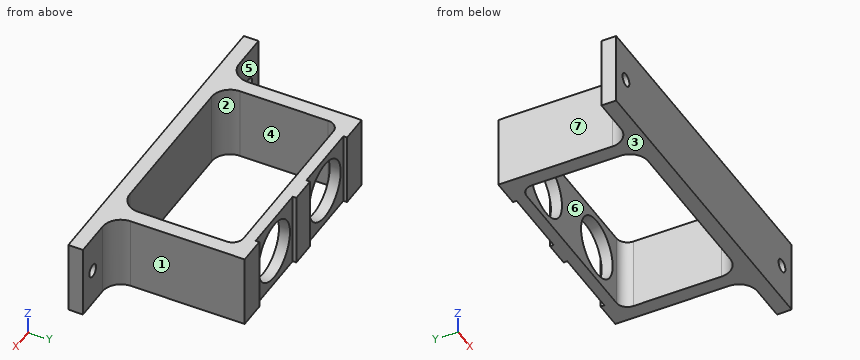
```python
from build123d import *

# Parameters (mm, degrees)
SKETCH_1_W          = 90
SKETCH_1_H          = 20
SKETCH_1_R          = 1.75
EXTRUDE_1_DEPTH     = 4
SKETCH_2_W          = 4
SKETCH_2_H          = 20
EXTRUDE_2_DEPTH     = 32
SKETCH_3_W          = 60
SKETCH_3_H          = 20
SKETCH_3_R          = 8.1
EXTRUDE_3_DEPTH     = 4
FILLET_1_R          = 5
FILLET_2_R          = 3
SKETCH_4_W          = 19
SKETCH_4_H          = 20
CUT_EXTRUDE_1_DEPTH = 1


with BuildPart() as part:
    # 草图1 → 凸台-拉伸1 (new body)
    with BuildSketch(Plane(origin=(0, 0, 0), x_dir=(1, 0, 0), z_dir=(0, 1, 0))):
        with Locations((45, 10)):
            Rectangle(SKETCH_1_W, SKETCH_1_H)
        with Locations(Location((85, 10, 0), (0, 0, 270))):
            Circle(SKETCH_1_R, mode=Mode.SUBTRACT)
        with Locations(Location((5, 10, 0), (0, 0, 90))):
            Circle(SKETCH_1_R, mode=Mode.SUBTRACT)
    extrude(amount=EXTRUDE_1_DEPTH)

    # 草图2 → 凸台-拉伸2 (add)
    with BuildSketch(Plane(origin=(0, 4, 0), x_dir=(1, 0, 0), z_dir=(0, 1, 0))):
        with Locations((17, 10)):
            Rectangle(SKETCH_2_W, SKETCH_2_H)
        with Locations((73, 10)):
            Rectangle(SKETCH_2_W, SKETCH_2_H)
    extrude(amount=EXTRUDE_2_DEPTH)

    # 草图3 → 凸台-拉伸3 (add)
    with BuildSketch(Plane(origin=(0, 36, 0), x_dir=(1, 0, 0), z_dir=(0, 1, 0))):
        with Locations((45, 10)):
            Rectangle(SKETCH_3_W, SKETCH_3_H)
        with Locations(Location((32, 10, 0), (0, 0, 270))):
            Circle(SKETCH_3_R, mode=Mode.SUBTRACT)
        with Locations(Location((58, 10, 0), (0, 0, 270))):
            Circle(SKETCH_3_R, mode=Mode.SUBTRACT)
    extrude(amount=EXTRUDE_3_DEPTH)

    # 圆角1
    fillet_1_edges = [part.edges().sort_by_distance(p)[0] for p in [
        (15, 4, -10),
        (19, 4, -10),
        (75, 4, -10),
        (71, 4, -10),
    ]]
    fillet(fillet_1_edges, radius=FILLET_1_R)

    # 圆角2
    fillet_2_edges = [part.edges().sort_by_distance(p)[0] for p in [
        (19, 36, -10),
        (71, 36, -10),
    ]]
    fillet(fillet_2_edges, radius=FILLET_2_R)

    # 草图4 → 切除-拉伸1 (cut)
    with BuildSketch(Plane(origin=(0, 40, 0), x_dir=(1, 0, 0), z_dir=(0, 1, 0))):
        with Locations((32, 10)):
            Rectangle(SKETCH_4_W, SKETCH_4_H)
        with Locations((58, 10)):
            Rectangle(SKETCH_4_W, SKETCH_4_H)
    extrude(amount=-CUT_EXTRUDE_1_DEPTH, mode=Mode.SUBTRACT)


solid = part.part
```
Geometry: final body of the model. Coordinates: model frame, mm. Face numbers are marked on the shaded views. A direction names the side the tool comes from. Coordinates: 2 decimals unless noted, no trailing zeros. Order: outer loops, then holes, each group sorted by start corner. A loop starts at its lowest first (then second) coordinate and runs counter-clockwise, first axis right, second up. Notation, with made-up numbers: (28, -22.75) -> (43, -22.75) arc R35 cw to (43, 14.25) -> close; hole circle Ø11 at (80, -10.5). An arc over 180 degrees is marked (long way). Use CSV: the item, a comma, the result in double quotes.
1) Section B-B on y = 32. Output: boundary loops of the cut face in (x, z).
Findings:
outline,"(15, -20) -> (19, -20) -> (19, 0) -> (15, 0) -> close; (71, -20) -> (75, -20) -> (75, 0) -> (71, 0) -> close"
2) Access query for the marked faces 1, 2 and 3. Directions: +Z, -Z, +X, -X, +Y, -Y. A direction counts if a zero-diameter tool reaches every point of the face in a straight line with its end or side. Return the directions, or none.
Findings:
face 1,"+Z, -Z, +X, +Y"
face 2,"+Z, -Z"
face 3,"-Z, +X, -X, +Y, -Y"
3) Mould query, pull axis Y, two halves, no side actions, for the marked faces 4, 5, 6 and 7. Classes: +Y half, -Y half, draft (parallel to the pull), parting line (faces both ways), or undercut.
Findings:
face 4,"undercut"
face 5,"+Y half"
face 6,"undercut"
face 7,"draft"
4) Pin query (flat end, axial travel): pin 1 Ø10 at (y, z) = (21, -6.5) entering from -X; pin 2 Ø5.5 at (x, z) = (28, -7) entering from +Y; pin 3 Ø6 at (y, z) = (30.5, -7) entering from +X. Return the tip coordinate at first contact, or that it passes through.
Findings:
pin 1,"stops at x = 15"
pin 2,"stops at y = 4"
pin 3,"stops at x = 75"
5) Section A-A on x = 5. Output: boundary loops of the cut face in (y, z), then the cut area to 3 significant figures.
Findings:
outline,"(0, -20) -> (4, -20) -> (4, -11.75) -> (0, -11.75) -> close; (0, -8.25) -> (4, -8.25) -> (4, 0) -> (0, 0) -> close"
area,"66.0 mm^2"
6) Section D-D on x = 32. Output: boundary loops of the cut face in (y, z).
Findings:
outline,"(0, -20) -> (4, -20) -> (4, 0) -> (0, 0) -> close; (36, -20) -> (39, -20) -> (39, -18.1) -> (36, -18.1) -> close; (36, -1.9) -> (39, -1.9) -> (39, 0) -> (36, 0) -> close"
7) Line query: line 1 (X direction, y = 37.9, z = -10); line 2 (X direction, y = 3, z = -10); line 3 (X direction, y = 20, z = -2.75). Output: solid intervals per line, ascending.
Findings:
line 1,"x = 15 to 23.9, 40.1 to 49.9, 66.1 to 75"
line 2,"x = 0 to 3.25, 6.75 to 83.25, 86.75 to 90"
line 3,"x = 15 to 19, 71 to 75"
